Geometry check sheet. Reference: drawing and pictorial views, mm from the part's lowest x, y, z. Coordinates: 2 decimals unless noted, no trailing zeros. Write each loop counter-clockwise with the first axis right and the second up, starting at its lowest first coordinate (ties: lowest second). Pieces come first, ordered by that corner, then holes.
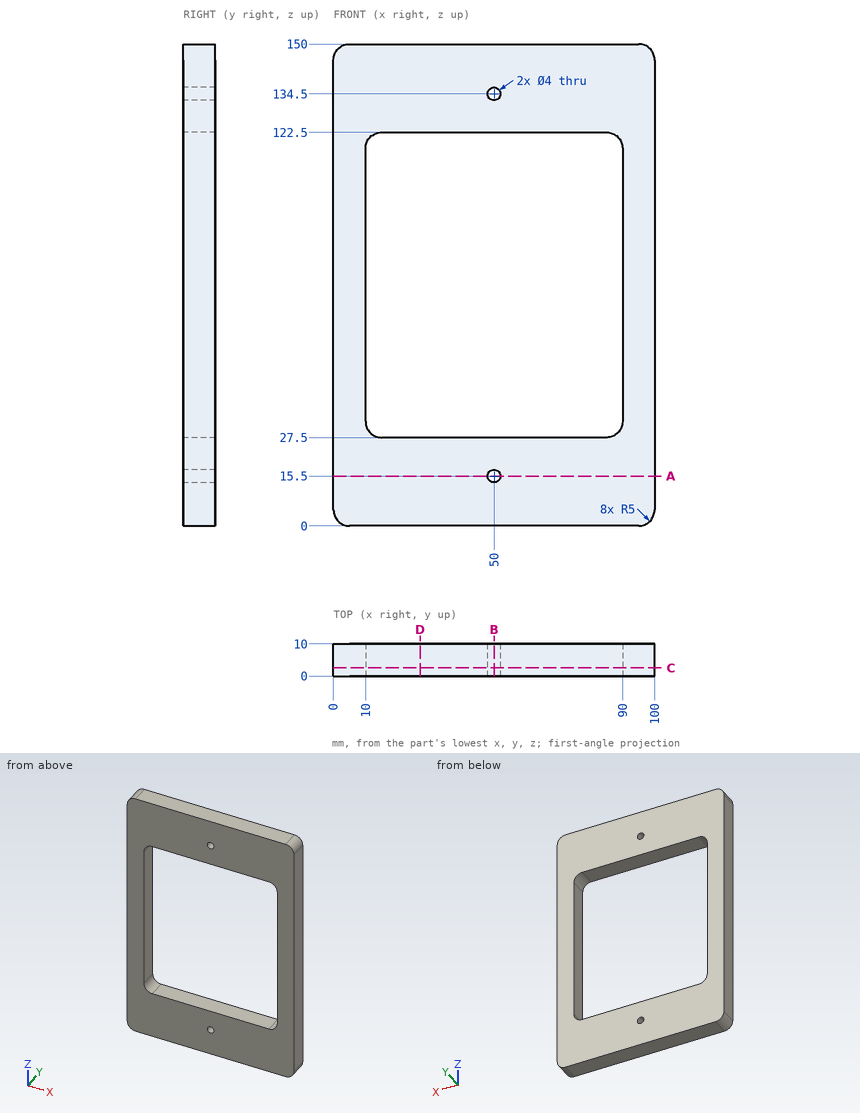
1. Sectioned sample at A-A, the plane z = 15.5. Record the boundary of the cut face in (x, y).
2. Sectioned sample at C-C, the plane y = 2.5. Record the boundary of the cut face in (x, z).
3. Gauge pin test, flat ends, axial feed: P1, Ø3, axis at x = 50, z = 134.5, coming from the +Y side; P2, Ø5, axis at y = 3, z = 62, coming from the -X side. Record the tip position at first contact, or that the pin passes through.
4. Material ranges on L1, parallel to Z at x = 50, y = 4.5; L2, parallel to X at y = 9.5, z = 69; L3, parallel to Z at x = 81.5, y = 1.5, recorded low to high.
5. Sectioned sample at D-D, the plane x = 27. Record the boundary of the cut face in (y, z).
6. Sectioned sample at B-B, the plane x = 50. Record the boundary of the cut face in (y, z), and give its area (3 significant figures).
Outcome:
1. outline: (0, 0) - (48, 0) - (48, 10) - (0, 10) - close; (52, 0) - (100, 0) - (100, 10) - (52, 10) - close
2. outline: (0, 5) arc R5 ccw to (5, 0) - (95, 0) arc R5 ccw to (100, 5) - (100, 145) arc R5 ccw to (95, 150) - (5, 150) arc R5 ccw to (0, 145) - close; hole (10, 32.5) arc R5 ccw to (15, 27.5) - (85, 27.5) arc R5 ccw to (90, 32.5) - (90, 117.5) arc R5 ccw to (85, 122.5) - (15, 122.5) arc R5 ccw to (10, 117.5) - close; hole circle Ø4 at (50, 15.5); hole circle Ø4 at (50, 134.5)
3. P1: passes through
3. P2: stops at x = 0
4. L1: z = 0 to 13.5, 17.5 to 27.5, 122.5 to 132.5, 136.5 to 150
4. L2: x = 0 to 10, 90 to 100
4. L3: z = 0 to 27.5, 122.5 to 150
5. outline: (0, 0) - (10, 0) - (10, 27.5) - (0, 27.5) - close; (0, 122.5) - (10, 122.5) - (10, 150) - (0, 150) - close
6. outline: (0, 0) - (10, 0) - (10, 13.5) - (0, 13.5) - close; (0, 17.5) - (10, 17.5) - (10, 27.5) - (0, 27.5) - close; (0, 122.5) - (10, 122.5) - (10, 132.5) - (0, 132.5) - close; (0, 136.5) - (10, 136.5) - (10, 150) - (0, 150) - close
6. area: 470 mm2
